Here's the drawing with two shaded views (mm, measured from the low corner). I have some questions. A direction names the side the tool comes from. Give positions to 0.01 mm unless a question says otherwise; leave off trailing zeros. Loops run counter-clockwise (first coordinate to the right, second up) from the corner with the lowest first, then second, coordinate; pieces in that order, holes last. Notation, with made-up numbers: (52, -17.5) -> (75, -17.5) arc R23 ccw to (75, -9.5) -> close; hole circle Ø4 at (-23.75, 8.5). An arc over 180 degrees is marked (long way). Write each question's results on one line, items separated by ' | '. Start each with the question number.
Q1. Will this pin go through, and if not, where does the flat tip stop? P1, Ø18, axis at x = 22, y = 11, coming from the +Z side.
Q2. If we section it at C-C, the plane x = 26.5: List the corners of the cut face in (y, z) for me, plus the area to 3 significant figures.
Q3. If we section it at B-B, the plane y = 21: List the corners of the cut face in (x, z) for me.
Q4. If I drill on line 1 along Y through (x, z) = (26.5, 2.4); line 2 along Y through (x, z) = (14.5, 1.15); line 3 along Y through (x, z) = (13.5, 1.75), over which ranges is the centre line in solid material (lowest first)?
Q5. Which directions (+Z, -Z, +X, -X, +Y, -Y) give clear straight access to the entire face, cutting with the end or side of a thin tool? Please do the marked faces 1 and 2.
Q6. If we section it at D-D, the plane y = 36: List the corners of the cut face in (x, z) for me.
Q7. If we section it at A-A, the plane x = 14.5: List the corners of the cut face in (y, z) for me.
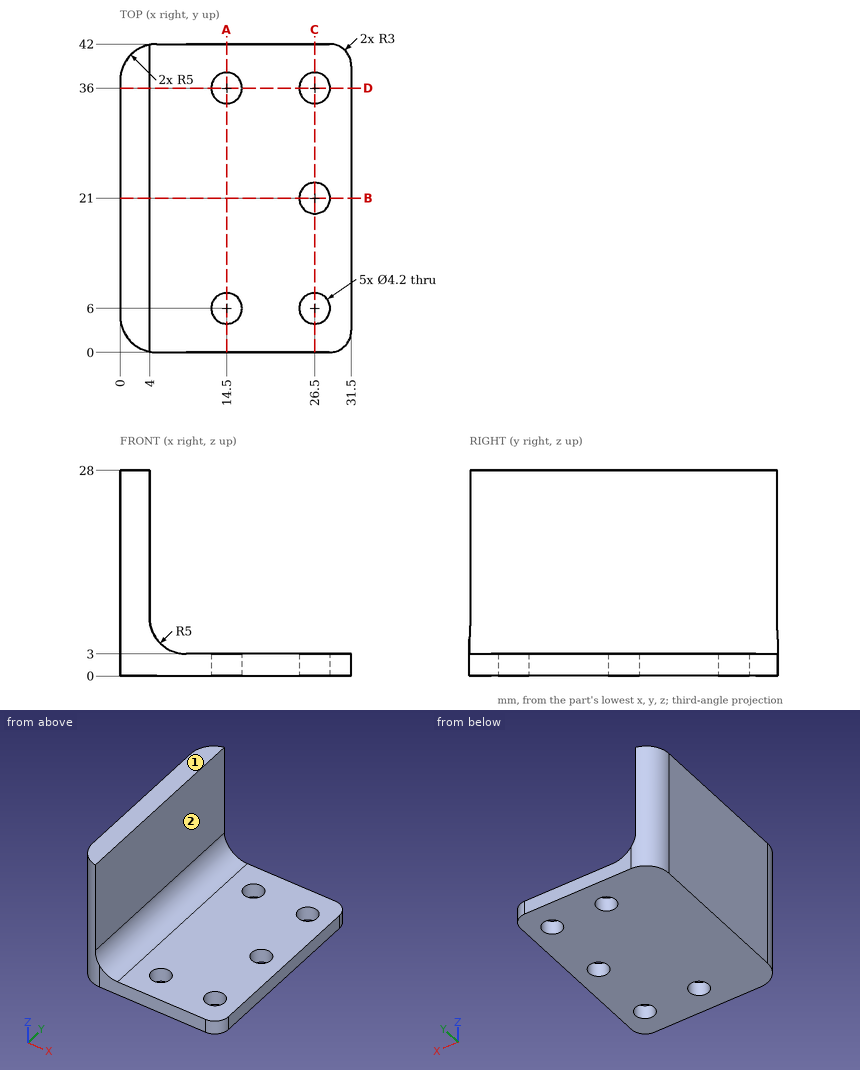
Final values:
1) P1: stops at z = 3
2) outline: (0, 0) -> (3.9, 0) -> (3.9, 3) -> (0, 3) -> close; (8.1, 0) -> (18.9, 0) -> (18.9, 3) -> (8.1, 3) -> close; (23.1, 0) -> (33.9, 0) -> (33.9, 3) -> (23.1, 3) -> close; (38.1, 0) -> (42, 0) -> (42, 3) -> (38.1, 3) -> close | area: 88.2 mm²
3) outline: (0, 0) -> (24.4, 0) -> (24.4, 3) -> (9, 3) arc R5 cw to (4, 8) -> (4, 28) -> (0, 28) -> close; (28.6, 0) -> (31.5, 0) -> (31.5, 3) -> (28.6, 3) -> close
4) line 1: y = 0 to 3.9, 8.1 to 18.9, 23.1 to 33.9, 38.1 to 42 | line 2: y = 0 to 3.9, 8.1 to 33.9, 38.1 to 42 | line 3: y = 0 to 4.15, 7.85 to 34.15, 37.85 to 42
5) face 1: +Z, +X, -X, +Y, -Y | face 2: +Z, +X, +Y, -Y
6) outline: (0, 0) -> (12.4, 0) -> (12.4, 3) -> (9, 3) arc R5 cw to (4, 8) -> (4, 28) -> (0, 28) -> close; (16.6, 0) -> (24.4, 0) -> (24.4, 3) -> (16.6, 3) -> close; (28.6, 0) -> (31.5, 0) -> (31.5, 3) -> (28.6, 3) -> close
7) outline: (0, 0) -> (3.9, 0) -> (3.9, 3) -> (0, 3) -> close; (8.1, 0) -> (33.9, 0) -> (33.9, 3) -> (8.1, 3) -> close; (38.1, 0) -> (42, 0) -> (42, 3) -> (38.1, 3) -> close
